For this review, take the finished solid that the model builds, in its own axes (mm). A direction names the side the tool comes from. Coordinates: 2 decimals unless noted, no trailing zeros. Order: outer loops, then holes, each group sorted by start corner. A loop starts at its lowest first (then second) coordinate and runs counter-clockwise, first axis right, second up.
from build123d import *

# Parameters (mm, degrees)
F0_W     = 24.638
F0_H     = 16.51
F1_DEPTH = 14.605
F2_W     = 12.211425
F2_H     = 10.16
F3_DEPTH = 24.13
F4_R     = 1.711361
F5_DEPTH = 25.4
F6_R     = 1.5621
F7_DEPTH = 25.4
F9_DEPTH = 0.127


with BuildPart() as f1:
    # F0 (on Front) → F1 (new body)
    with BuildSketch(Plane.XZ):
        with Locations((-0.772754, 5.392659)):
            Rectangle(F0_W, F0_H)
    extrude(amount=F1_DEPTH)

    # F2 (on face) → F3 (cut)
    with BuildSketch(Plane(origin=(-13.091754, 0, 0), x_dir=(0, -1, 0), z_dir=(-1, 0, 0))):
        with Locations((7.292173, 7.007426)):
            Rectangle(F2_W, F2_H)
    extrude(amount=-F3_DEPTH, mode=Mode.SUBTRACT)

    # F4 (on face) → F5 (cut)
    with BuildSketch(Plane(origin=(11.038246, 0, 0), x_dir=(0, -1, 0), z_dir=(-1, 0, 0))):
        with Locations((7.292174, 7.007426)):
            Circle(F4_R)
    extrude(amount=-F5_DEPTH, mode=Mode.SUBTRACT)

    # F6 (on face) → F7 (cut)
    with BuildSketch(Plane.YZ.offset(11.546246)):
        with Locations((-2.5984, -0.579538)):
            Circle(F6_R)
        with Locations((-12.017213, -0.579538)):
            Circle(F6_R)
    extrude(amount=-F7_DEPTH, mode=Mode.SUBTRACT)

    # F8 (on face) → F9 (join)
    with BuildSketch(Plane(origin=(0, 0, -2.862341), x_dir=(1, 0, 0), z_dir=(0, 0, -1))):
        with BuildLine():
            Line((7.308862, 8.876015), (7.006992, 9.298633))
            ThreePointArc((7.006992, 9.298633), (5.738039, 7.660322), (6.644748, 5.796942))
            ThreePointArc((6.644748, 5.796942), (7.851761, 5.628954), (8.74961, 6.45295))
            ThreePointArc((8.74961, 6.45295), (8.365962, 7.347122), (7.39537, 7.278706))
            Line((7.39537, 7.278706), (7.477945, 6.793113))
            ThreePointArc((7.477945, 6.793113), (7.861302, 7.000267), (8.244659, 6.793113))
            ThreePointArc((8.244659, 6.793113), (7.849436, 6.179211), (7.127739, 6.068625))
            ThreePointArc((7.127739, 6.068625), (6.293176, 7.532006), (7.308862, 8.876015))
        make_face()
    extrude(amount=F9_DEPTH)


solid = f1.part
1. Take a section at C-C, the plane x = 4. Give the boundary of the cut face in (y, z) (3 decimals), plus the area to 3 significant figures.
Answer below:
outline: (-14.605, -2.862) - (0, -2.862) - (0, 13.648) - (-14.605, 13.648) - close; hole circle Ø3.124 at (-12.017, -0.58); hole (-13.398, 1.927) - (-1.186, 1.927) - (-1.186, 12.087) - (-13.398, 12.087) - close; hole circle Ø3.124 at (-2.598, -0.58)
area: 102 mm2
2. Clearance check with flat-ended pins moving along their axes: pin 1 Ø3.5 at (x, y) = (-1.5, -7) entering from -Z; pin 2 Ø4.5 at (y, z) = (-7.29, 7.01) entering from -X. State where each tip first meets the part, or that it passes through.
Answer below:
pin 1: stops at z = -2.86
pin 2: stops at x = 11.04
3. Machinability: for faces 1 (the face through (-0.6, -4.16, -0.51)), 2 (the face through (-1, -1.186, 7)), which of the approach directions +Z, -Z, +X, -X, +Y, -Y give a long, thin tool a straight path to every point of the face, cutting with its end or side? Answer none if there is none.
Answer below:
face 1: +X, -X
face 2: -X
4. Take a section at A-A, the plane z = 3.75. Give the boundary of the cut face in (x, y) (3 decimals), plus the area to 3 significant figures.
Answer below:
outline: (-13.092, -14.605) - (11.546, -14.605) - (11.546, 0) - (-13.092, 0) - (-13.092, -1.186) - (11.038, -1.186) - (11.038, -13.398) - (-13.092, -13.398) - close
area: 65.2 mm2
5. The part is to be moulded in two halves that separate along Y. For faces 3 (the face through (-1, -7, 1.927)), 4 (the face through (7.7, -7.2, -2.989)), 5 (the face through (-1, -14.605, 6)), 6 (the face through (-1, 0, 6)), say which applies: +Y half, -Y half, draft (parallel to the pull), parting line (faces both ways), or undercut.
Answer below:
face 3: undercut
face 4: draft
face 5: -Y half
face 6: +Y half
6. Take a section at D-D, the plane y = -3.5. Give the boundary of the cut face in (x, z), plus the area to 3 significant figures.
Answer below:
outline: (-13.09, -2.86) - (11.55, -2.86) - (11.55, -1.86) - (-13.09, -1.86) - close; (-13.09, 0.7) - (11.55, 0.7) - (11.55, 13.65) - (-13.09, 13.65) - (-13.09, 12.09) - (11.04, 12.09) - (11.04, 1.93) - (-13.09, 1.93) - close
area: 98.8 mm2
7. To check wall thickness, follow L1, parallel to Y at x = -5.25, z = -0.5 (3 decimals); L2, parallel to Z at x = 8.75, y = -4.5; L3, parallel to Y at x = 2.25, z = 2 (3 decimals). State the ranges of each line that lie inside material, in increasing order.
Answer below:
L1: y = -14.605 to -13.577, -10.457 to -4.158, -1.038 to 0
L2: z = -2.86 to 1.93, 12.09 to 13.65
L3: y = -14.605 to -13.398, -1.186 to 0
8. Take a section at B-B, the plane y = -12. Give the boundary of the cut face in (x, z), plus the area to 3 significant figures.
Answer below:
outline: (-13.09, -2.86) - (11.55, -2.86) - (11.55, -2.14) - (-13.09, -2.14) - close; (-13.09, 0.98) - (11.55, 0.98) - (11.55, 13.65) - (-13.09, 13.65) - (-13.09, 12.09) - (11.04, 12.09) - (11.04, 1.93) - (-13.09, 1.93) - close
area: 84.6 mm2
